```python
from build123d import *

# Parameters (mm, degrees)
FILLET1_R          = 0.762
SKETCH2_R          = 3.175
CUT_EXTRUDE1_DEPTH = 21.59


# Read off the part's stored shape, not the designer's step: Shell1
with BuildPart() as part:
    # Sketch1 → Revolve1 (revolve)
    with BuildSketch(Plane.XY, mode=Mode.PRIVATE) as revolve1_sk:
        Polygon((19.6723, 0), (19.6723, 1.778), (17.6403, 1.778), (17.6403, 4.4958), (19.6723, 4.4958), (19.6723, 5.7658), (16.9545, 5.7658), (20.4978, 21.844), (20.4978, 24.892), (0, 24.892), (0, 0), align=None)
    revolve(revolve1_sk.sketch.rotate(Axis((0, 0, 0), (0, 1, 0)), 90), axis=Axis((0, 0, 0), (0, 1, 0)))

    # Fillet1
    fillet1_edges = [part.edges().sort_by_distance(p)[0] for p in [
        (0, 0, 19.6723),
    ]]
    fillet(fillet1_edges, radius=FILLET1_R)

    # Shell1 outline → Shell1 (revolve, cut)
    with BuildSketch(Plane.XY):
        Polygon((16.4465, 4.572), (15.468965439, 4.572), (19.304, 21.973984782), (19.304, 24.892), (0, 24.892), (0, 0), (18.4785, 0), (18.4785, 0.5842), (16.4465, 0.5842), align=None)
    revolve(axis=Axis((0, 0, 0), (0, 1, 0)), mode=Mode.SUBTRACT)

    # Sketch2 → Cut-Extrude1 (cut, symmetric)
    with BuildSketch(Plane.XY):
        with Locations(Location((0, 13.843, 0), (0, 0, 270.000000005))):
            Circle(SKETCH2_R)
        with Locations(Location((-9.533032066, 13.843, 0), (0, 0, 215.10740663))):
            Circle(SKETCH2_R)
        with Locations(Location((9.525, 13.843, 0), (0, 0, 247.150680843))):
            Circle(SKETCH2_R)
    extrude(amount=CUT_EXTRUDE1_DEPTH, both=True, mode=Mode.SUBTRACT)


solid = part.part
```
Input: part model. Units: mm. Frame: model coordinates. A direction names the side the tool comes from. Round coordinates to 2 decimals unless told otherwise and drop trailing zeros. Loops run counter-clockwise (first coordinate to the right, second up) from the corner with the lowest first, then second, coordinate; pieces in that order, holes last. Notation, with made-up numbers: (-23, 41.5) - (-18, 41.5) arc R16 ccw to (-18, 60.5) - close; hole circle Ø8 at (-5.75, 33). An arc over 180 degrees is marked (long way). One line per item, written item: value. Start each with the question number.
(1) Section D-D, the plane y = 16. Return loops of the section in (x, z).
(2) Ray query, line 1 (X direction, y = 2.5, z = 0); line 2 (Z direction, x = 1.5, y = 23); line 3 (Z direction, x = -11, y = 10.25). Return the intervals inside material, ascending. Write a range as [from, to].
(3) Contact query for flat-ended pins moving along their axis: P1, Ø4, axis at x = 9.525, y = 13.843, coming from the -Z side; P2, Ø7.5, axis at x = 9.525, y = 13.843, coming from the -Z side; P3, Ø12, axis at y = 5.5, z = 4.5, coming from the +X side; P4, Ø4, axis at x = 15.5, y = 14, coming from the +Z side. Output: stop coordinate, or through.
(4) Section B-B, the plane y = 13. Return loops of the section in (x, z).
(5) Access query for faces 1 (the cylindrical face through (-2.41, 0.3, -18.32)), 2 (the cylindrical face through (12.47, 23.39, 16.27)), 3 (the cylindrical face through (-15.319, 23.453, 11.746)), 4 (the flat face through (-18, 4.496, -3)). Directions: +Z, -Z, +X, -X, +Y, -Y. A direction counts if a zero-diameter tool reaches every point of the face in a straight line with its end or side. Return the directions, or none.
(6) Section C-C, the plane x = 11.5. Count the separate pieces of the cut face and the enclosed holes in it, plus the area to 3 significant figures.
(7) Draft query along Y for faces 5 (the cylindrical face through (11.97, 1.28, 15.61)), 6 (the flat face through (-17, 0.584, 1)), 7 (the cylindrical face through (2.68, 12.14, 17.81)). Return one class per face: +Y half, -Y half, draft (parallel to the pull), parting line (faces both ways), or undercut.
Results below:
1. outline: (-11.86, -15.11) - (-11.86, -13.52) arc R17.99 cw to (-11.86, 13.52) - (-11.86, 15.11) arc R19.21 ccw to start; (-7.2, -17.81) arc R19.21 ccw to (-2.33, -19.07) - (-2.33, -17.84) arc R17.99 cw to (-7.2, -16.48) - close; (-7.2, 16.48) arc R17.99 cw to (-2.33, 17.84) - (-2.33, 19.07) arc R19.21 ccw to (-7.2, 17.81) - close; (2.33, -19.07) arc R19.21 ccw to (7.2, -17.81) - (7.2, -16.49) arc R17.99 cw to (2.33, -17.84) - close; (2.33, 17.84) arc R17.99 cw to (7.2, 16.49) - (7.2, 17.81) arc R19.21 ccw to (2.33, 19.07) - close; (11.85, -15.12) arc R19.21 ccw to (11.85, 15.12) - (11.85, 13.53) arc R17.99 cw to (11.85, -13.53) - close
2. line 1: [-17.64, -16.45], [16.45, 17.64]
2. line 2: [-20.44, -19.25], [19.25, 20.44]
2. line 3: [-14.18, -12.59], [12.59, 14.18]
3. P1: through
3. P2: z = -18.09
3. P3: x = 19.67
3. P4: z = 13.13
4. outline: (-12.59, -13.62) - (-12.59, -11.9) arc R17.33 cw to (-12.59, 11.9) - (-12.59, 13.62) arc R18.55 ccw to start; (-6.47, -17.38) arc R18.55 ccw to (-3.06, -18.29) - (-3.06, -17.05) arc R17.33 cw to (-6.47, -16.07) - close; (-6.47, 16.07) arc R17.33 cw to (-3.06, 17.05) - (-3.06, 18.29) arc R18.55 ccw to (-6.47, 17.38) - close; (3.06, -18.29) arc R18.55 ccw to (6.46, -17.39) - (6.46, -16.08) arc R17.33 cw to (3.06, -17.05) - close; (3.06, 17.05) arc R17.33 cw to (6.46, 16.08) - (6.46, 17.39) arc R18.55 ccw to (3.06, 18.29) - close; (12.59, -13.63) arc R18.55 ccw to (12.59, 13.63) - (12.59, 11.91) arc R17.33 cw to (12.59, -11.91) - close
5. face 1: -Y
5. face 2: +Y, -Y
5. face 3: +Y
5. face 4: none
6. separate pieces: 4
6. enclosed holes: 0
6. area: 78.2 mm^2
7. face 5: draft
7. face 6: -Y half
7. face 7: undercut
